For this review, take the finished solid that the model builds, in its own axes (mm). Coordinates: 2 decimals unless noted, no trailing zeros. Write each loop counter-clockwise with the first axis right and the second up, starting at its lowest first coordinate (ties: lowest second). Pieces come first, ordered by that corner, then holes.
1) We need section D-D on z = -18.5. Write out the cut boundary in (x, y), then the cut area to 3 significant figures.
2) Mouldability with a two-part tool opening along Z and no side actions: class faces 1 (the face through (-1, 0, 8)), 2 (the face through (-35, 6, -38.1)), 3 (the face through (-1, 6, 38.1)), 4 (the face through (-18.91, 6.44, 15.88)) as pulls with the +Z half, pulls with the -Z half, needs draft (parallel to the pull), parting line crosses it, or undercut.
3) We need section C-C on y = 5.75. Write out the cut boundary in (x, z) (3 decimals).
4) To check wall thickness, follow line 1 along X through (y, z) = (8.5, 19.05) (3 decimals); line 2 along X through (y, z) = (0.75, 18); line 3 along Z through (x, y) = (19.05, 6.5) (3 decimals). State the ranges of each line that lie inside material, in increasing order.
5) We need section B-B on x = -19.05. Write out the cut boundary in (y, z) (3 decimals), then the cut area to 3 significant figures.
6) We need section A-A on z = 19.05. Write out the cut boundary in (x, y) (3 decimals).
from build123d import *

# Parameters (mm, degrees)
BOSS_EXTRUDE1_DEPTH = 12.7
SKETCH2_R           = 3.175
CUT_EXTRUDE1_DEPTH  = 12.7


with BuildPart() as part:
    # Sketch1 → Boss-Extrude1 (new body)
    with BuildSketch(Plane(origin=(0, 0, 0), x_dir=(1, 0, 0), z_dir=(0, 1, 0))):
        with BuildLine():
            Line((38.1, 38.1), (32.534068682, 38.1))
            ThreePointArc((32.534068682, 38.1), (0, 15.875), (-32.534068682, 38.1))
            Line((-32.534068682, 38.1), (-38.1, 38.1))
            Line((-38.1, 38.1), (-38.1, -38.1))
            Line((-38.1, -38.1), (38.1, -38.1))
            Line((38.1, -38.1), (38.1, 38.1))
        make_face()
    extrude(amount=BOSS_EXTRUDE1_DEPTH)

    # Sketch2 → Cut-Extrude1 (cut)
    with BuildSketch(Plane(origin=(0, 12.7, 0), x_dir=(1, 0, 0), z_dir=(0, 1, 0))):
        with Locations(Location((-19.05, -19.05, 0), (0, 0, 270))):
            Circle(SKETCH2_R)
        with Locations(Location((19.05, -19.05, 0), (0, 0, 90))):
            Circle(SKETCH2_R)
    extrude(amount=-CUT_EXTRUDE1_DEPTH, mode=Mode.SUBTRACT)


solid = part.part
Result:
1. outline: (-38.1, 0) - (-13.28, 0) - (-13.28, 12.7) - (-38.1, 12.7) - close; (13.28, 0) - (38.1, 0) - (38.1, 12.7) - (13.28, 12.7) - close
1. area: 630 mm2
2. face 1: needs draft
2. face 2: pulls with the -Z half
2. face 3: pulls with the +Z half
2. face 4: undercut
3. outline: (-38.1, -38.1) - (-32.534, -38.1) arc R34.925 cw to (32.534, -38.1) - (38.1, -38.1) - (38.1, 38.1) - (-38.1, 38.1) - close; hole circle Ø6.35 at (-19.05, 19.05); hole circle Ø6.35 at (19.05, 19.05)
4. line 1: x = -38.1 to -22.225, -15.875 to 15.875, 22.225 to 38.1
4. line 2: x = -38.1 to -22.05, -16.05 to 16.05, 22.05 to 38.1
4. line 3: z = -21.528 to 15.875, 22.225 to 38.1
5. outline: (0, -21.528) - (12.7, -21.528) - (12.7, 15.875) - (0, 15.875) - close; (0, 22.225) - (12.7, 22.225) - (12.7, 38.1) - (0, 38.1) - close
5. area: 677 mm2
6. outline: (-38.1, 0) - (-22.225, 0) - (-22.225, 12.7) - (-38.1, 12.7) - close; (-15.875, 0) - (15.875, 0) - (15.875, 12.7) - (-15.875, 12.7) - close; (22.225, 0) - (38.1, 0) - (38.1, 12.7) - (22.225, 12.7) - close
